```python
from build123d import *

# Parameters (mm, degrees)
BOSS_EXTRUDE1_DEPTH     = 6.5
BOSS_EXTRUDE2_DEPTH     = 2
CUT_EXTRUDE1_DEPTH      = 20.059283612
CUT_EXTRUDE1_DEPTH_BACK = 20.059283612
CHAMFER1_SIZE           = 0.4


with BuildPart() as part:
    # Sketch1 → Boss-Extrude1 (new body)
    with BuildSketch(Plane.XY):
        Polygon((0, -6.142777017), (2.175697935, -3.768419365), (5.319800946, -3.071388508), (4.351395869, 0), (5.319800946, 3.071388508), (2.175697935, 3.768419365), (0, 6.142777017), (-2.175697935, 3.768419365), (-5.319800946, 3.071388508), (-4.351395869, 0), (-5.319800946, -3.071388508), (-2.175697935, -3.768419365), align=None)
    extrude(amount=-BOSS_EXTRUDE1_DEPTH)

    # Sketch2 → Boss-Extrude2 (add)
    # profile 1 of 2: a face of its own
    with BuildSketch(Plane.XY):
        Polygon((9.594041495, 0), (11.729199677, 6.771856591), (4.797020748, 8.30868366), (0, 13.543713181), (-4.797020748, 8.30868366), (-11.729199677, 6.771856591), (-9.594041495, 0), (-11.729199677, -6.771856591), (-4.797020748, -8.30868366), (0, -13.543713181), (4.797020748, -8.30868366), (11.729199677, -6.771856591), align=None)
        Polygon((5.319800946, -3.071388508), (4.351395869, 0), (5.319800946, 3.071388508), (2.175697935, 3.768419365), (0, 6.142777017), (-2.175697935, 3.768419365), (-5.319800946, 3.071388508), (-4.351395869, 0), (-5.319800946, -3.071388508), (-2.175697935, -3.768419365), (0, -6.142777017), (2.175697935, -3.768419365), align=None, mode=Mode.SUBTRACT)
    # profile 2 of 2: a face of its own
    with BuildSketch(Plane.XY):
        Polygon((2.175697935, -3.768419365), (5.319800946, -3.071388508), (4.351395869, 0), (5.319800946, 3.071388508), (2.175697935, 3.768419365), (0, 6.142777017), (-2.175697935, 3.768419365), (-5.319800946, 3.071388508), (-4.351395869, 0), (-5.319800946, -3.071388508), (-2.175697935, -3.768419365), (0, -6.142777017), align=None)
    extrude(amount=BOSS_EXTRUDE2_DEPTH)

    # Sketch1_4 → Cut-Extrude1 (cut, two sides: drawn at the far end of the back side and taken through both)
    with BuildSketch(Plane.XY.offset(-CUT_EXTRUDE1_DEPTH_BACK)):
        with BuildLine():
            ThreePointArc((1.15, 0), (0.813172798, 0.813172798), (0, 1.15))
            Line((0, 1.15), (0, -1.15))
            ThreePointArc((0, -1.15), (0.813172798, -0.813172798), (1.15, 0))
        make_face()
        with BuildLine():
            Line((0, -1.15), (0, 1.15))
            ThreePointArc((0, 1.15), (-1.15, 0), (0, -1.15))
        make_face()
    extrude(amount=CUT_EXTRUDE1_DEPTH + CUT_EXTRUDE1_DEPTH_BACK, mode=Mode.SUBTRACT)

    # Chamfer1
    chamfer1_edges = [part.edges().sort_by_distance(p)[0] for p in [
        (3.74774944, -3.419903937, 0),
        (1.087848967, -4.955598191, 0),
        (-1.087848967, -4.955598191, 0),
        (-3.74774944, -3.419903937, 0),
        (-4.835598408, -1.535694254, 0),
        (-4.835598408, 1.535694254, 0),
        (-3.74774944, 3.419903937, 0),
        (-1.087848967, 4.955598191, 0),
        (1.087848967, 4.955598191, 0),
        (3.74774944, 3.419903937, 0),
        (4.835598408, 1.535694254, 0),
        (4.835598408, -1.535694254, 0),
    ]]
    chamfer(chamfer1_edges, length=CHAMFER1_SIZE)


solid = part.part
```
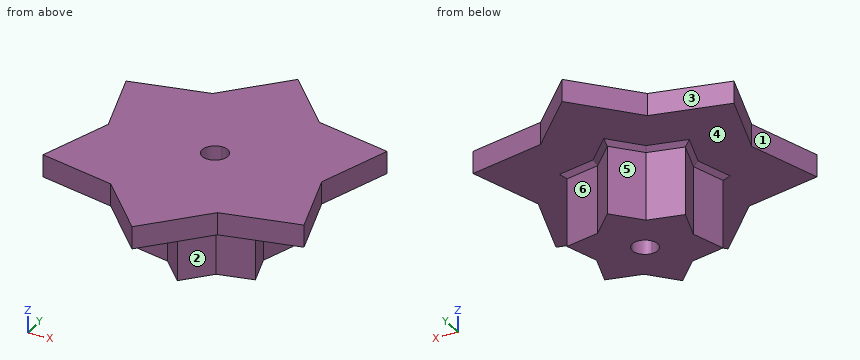
Part model, mm, in its own coordinate system. Face numbers are marked on the shaded views. A direction names the side the tool comes from. Give positions to 0.01 mm unless a question says otherwise; leave off trailing zeros. Order: outer loops, then holes, each group sorted by start corner. A loop starts at its lowest first (then second) coordinate and runs counter-clockwise, first axis right, second up. Notation, with made-up numbers: M -5.75,-14.75 L 12.25,-14.75 A16 ccw 12.25,1.25 Z; hole C -37,37.25 d8. An arc over 180 degrees is marked long. Use a Markdown table: item, result. Add a question column.
(1) Drop flat-ended pins along their axis: P1, Ø2, axis at y = 3, z = 1, coming from the +X side; P2, Ø4, axis at y = 7.5, z = -5.5, coming from the +X side; P3, Ø1.5, axis at x = -1.5, z = -1, coming from the +Y side. Give the stop position or say it passes through.
(2) Probe line 1 along Z through (x, y) = (7.5, -2); line 2 along X through (y, z) = (-1, -1.25); line 3 along Y through (x, z) = (9, 1.25). List the from-to ranges inside material, lowest first. Write a range as [from, to].
(3) Saw through at A-A, the plane z = -3.5. Give the cut face in (x, y), and give its area (3 significant figures).
(4) Saw through at C-C, the plane y = -4.5. Give the cut face in (x, z).
(5) Saw through at D-D, the plane z = 1.25. Give the cut face in (x, y), and give its area (3 significant figures).
(6) Mould opens along Y. For the marked faces 1, 2 and 3 say: +Y half, -Y half, draft (parallel to the pull), parting line (faces both ways), or undercut.
(7) Saw through at B-B, the plane x = -1.5. Give the cut face in (y, z), and give its area (3 significant figures).
(8) 3-axis set-ups, long thin cutter, end or side, ignore diameter. For the marked faces 4, 5 and 6: which of +Z, -Z, +X, -X, +Y, -Y reach the whole face in a straight line?
Answer key:
| question | item | result |
|---|---|---|
| 1 | P1 | x = 10.86 |
| 1 | P2 | x = 0.59 |
| 1 | P3 | y = 5.32 |
| 2 | line 1 | [0, 2] |
| 2 | line 2 | [-4.67, -0.57], [0.57, 4.67] |
| 2 | line 3 | [-7.38, 7.38] |
| 3 | outline | M -5.32,-3.07 L -2.18,-3.77 L 0,-6.14 L 2.18,-3.77 L 5.32,-3.07 L 4.35,0 L 5.32,3.07 L 2.18,3.77 L 0,6.14 L -2.18,3.77 L -5.32,3.07 L -4.35,0 Z; hole C 0,0 d2.3 |
| 3 | area | 76.0 mm^2 |
| 4 | outline | M -11.01,0 L -2.05,0 L -1.51,-0.4 L -1.51,-6.5 L 1.51,-6.5 L 1.51,-0.4 L 2.05,0 L 11.01,0 L 11.01,2 L -11.01,2 Z |
| 5 | outline | M -11.73,-6.77 L -4.8,-8.31 L 0,-13.54 L 4.8,-8.31 L 11.73,-6.77 L 9.59,0 L 11.73,6.77 L 4.8,8.31 L 0,13.54 L -4.8,8.31 L -11.73,6.77 L -9.59,0 Z; hole C 0,0 d2.3 |
| 5 | area | 386 mm^2 |
| 6 | face 1 | undercut |
| 6 | face 2 | -Y half |
| 6 | face 3 | +Y half |
| 7 | outline | M -11.91,0 L -5.1,0 L -4.51,-0.4 L -4.51,-6.5 L 4.51,-6.5 L 4.51,-0.4 L 5.1,0 L 11.91,0 L 11.91,2 L -11.91,2 Z |
| 7 | area | 106 mm^2 |
| 8 | face 4 | -Z |
| 8 | face 5 | -Z, -X, +Y |
| 8 | face 6 | -Z, +X, +Y |
